Source: CAD feature listing. Evaluate the final solid. Frame: model axes, mm. A direction names the side the tool comes from. Round coordinates to 2 decimals unless told otherwise and drop trailing zeros. Loops run counter-clockwise (first coordinate to the right, second up) from the corner with the lowest first, then second, coordinate; pieces in that order, holes last. Notation, with made-up numbers: (80, -29.5) -> (88, -29.5) arc R17 ccw to (88, 2.5) -> close; hole circle Ø6 at (-29.75, 8). An arc over 180 degrees is marked (long way). Put each result on its own line as item: value. Start each with the question number.
1. Cut plane D-D (y = 216.5). Return the cut outline in (x, z) (3 decimals), then the cut area to 3 significant figures.
2. Set-up query: faces 1 (the flat face through (-104.51, 109.14, 1.57)), 2 (the flat face through (-156.49, 73.08, 1.57)). Return all of +Z, -Z, +X, -X, +Y, -Y with unobstructed straight access to the full face (end or side cutting, diameter ignored); none if empty.
3. Cut plane A-A (y = 186). Return the cut outline in (x, z) (3 decimals), then the cut area to 3 significant figures.
4. Cut plane C-C (x = -72.5). Return the cut outline in (y, z) (3 decimals), then the cut area to 3 significant figures.
5. Contact query for flat-ended pins moving along their axis: pin 1 (1.5 mm diameter, centred on x = 101, z = 1.5, fed in from +Y); pin 2 (1.7 mm diameter, centred on y = 231.5, z = 1.5, fed in from +X); pin 3 (1.6 mm diameter, centred on x = -182, z = 1.5, fed in from -Y). Output: stop coordinate, or through.
6. Material intervals for L1, parallel to X at y = 112.5, z = 0.85; L2, parallel to X at y = 188, z = 1.8; L3, parallel to Y at x = -52.5, z = 0.5, sorted ascending.
7. Cut plane B-B (y = 133). Return the cut outline in (x, z) (3 decimals).
```python
from build123d import *

# Parameters (mm, degrees)
BOSS_EXTRUDE1_DEPTH = 3.175
FILLET1_R           = 12.7
SKETCH3_W           = 50.8
SKETCH3_H           = 1.5875
BOSS_EXTRUDE2_DEPTH = 3.175
CUT_EXTRUDE1_DEPTH  = 305.700701144
CUT_EXTRUDE2_DEPTH  = 305.700701144
CUT_EXTRUDE3_REACH  = 306.045
SKETCH6_W           = 3.175
SKETCH6_H           = 11.1125
CUT_EXTRUDE5_START  = -3.175
CUT_EXTRUDE5_DEPTH  = 3.175
SKETCH8_W           = 471.002245988
SKETCH8_H           = 22.673608405
CUT_EXTRUDE6_DEPTH  = 305.045309672


with BuildPart() as part:
    # Sketch1 → Boss-Extrude1 (new body)
    with BuildSketch(Plane.XY):
        Polygon((-196.85, 0), (-63.5, 230.968975189), (63.5, 230.968975189), (196.85, 0), (167.520606325, 0), (48.835303163, 205.568975189), (-48.835303163, 205.568975189), (-167.520606325, 0), align=None)
    extrude(amount=BOSS_EXTRUDE1_DEPTH)

    # Fillet1
    fillet1_edges = [part.edges().sort_by_distance(p)[0] for p in [
        (167.520606325, 0, 1.5875),
        (48.835303163, 205.568975189, 1.5875),
        (-48.835303163, 205.568975189, 1.5875),
        (-167.520606325, 0, 1.5875),
    ]]
    fillet(fillet1_edges, radius=FILLET1_R)

    # Sketch3 → Boss-Extrude2 (add)
    with BuildSketch(Plane(origin=(0, 0, 0), x_dir=(-1, 0, 0), z_dir=(0, 0, -1))):
        Polygon((81.638815329, 202.726625451), (80.264, 201.932875451), (105.664, 157.938784939), (107.038815329, 158.732534939), align=None)
        Polygon((143.614815329, 95.381044601), (142.24, 94.587294601), (167.64, 50.593204089), (169.014815329, 51.386954089), align=None)
        with Locations((0, 231.762725189)):
            Rectangle(SKETCH3_W, SKETCH3_H)
    boss_extrude2 = extrude(amount=-BOSS_EXTRUDE2_DEPTH)

    # Sketch5 → Cut-Extrude1 (cut, through all)
    with BuildSketch(Plane(origin=(0, 0, 0), x_dir=(-1, 0, 0), z_dir=(0, 0, -1))):
        Polygon((-175.966912895, 19.672783942), (-185.491912895, 19.672783942), (-187.325, 16.497783942), (-186.309, 16.497783942), (-175.966912895, 16.497783942), align=None)
        Polygon((-186.309, 16.497783942), (-187.325, 16.497783942), (-196.85, 0), (-195.834, 0), align=None)
        Polygon((-121.132358029, 112.096802923), (-129.38125, 116.859302923), (-130.96875, 114.109672266), (-122.719858029, 109.347172266), align=None)
    cut_extrude1 = extrude(amount=-CUT_EXTRUDE1_DEPTH, mode=Mode.SUBTRACT)

    # Sketch4 → Cut-Extrude2 (cut, through all)
    with BuildSketch(Plane(origin=(0, 0, 0), x_dir=(-1, 0, 0), z_dir=(0, 0, -1))):
        Polygon((-61.666912895, 230.968975189), (-56.904412895, 222.720083218), (-59.654043552, 221.132583218), (-64.416543552, 229.381475189), (-63.5, 230.968975189), align=None)
    cut_extrude2 = extrude(amount=-CUT_EXTRUDE2_DEPTH, mode=Mode.SUBTRACT)

    # Mirror1: Boss-Extrude2, Cut-Extrude1, Cut-Extrude2 across plane
    add(boss_extrude2.mirror(Plane(origin=(0, 0, 0), x_dir=(0, 0, 1), z_dir=(1, 0, 0))))
    add(cut_extrude1.mirror(Plane(origin=(0, 0, 0), x_dir=(0, 0, 1), z_dir=(1, 0, 0))), mode=Mode.SUBTRACT)
    add(cut_extrude2.mirror(Plane(origin=(0, 0, 0), x_dir=(0, 0, 1), z_dir=(1, 0, 0))), mode=Mode.SUBTRACT)

    # Sketch6 → Cut-Extrude3 (cut, up to next)
    with BuildSketch(Plane(origin=(0, 0, 0), x_dir=(-1, 0, 0), z_dir=(0, 0, -1)), mode=Mode.PRIVATE) as cut_extrude3_sk1:
        with Locations((0, 227.000225189)):
            Rectangle(SKETCH6_W, SKETCH6_H)
    cut_extrude3_tool1 = extrude(cut_extrude3_sk1.sketch, amount=-CUT_EXTRUDE3_REACH, mode=Mode.PRIVATE) & part.part
    add(cut_extrude3_tool1.solids().sort_by_distance((0, 227.000225, 0))[0], mode=Mode.SUBTRACT)

    # Sketch7 → Cut-Extrude5 (cut)
    with BuildSketch(Plane(origin=(0, 0, 0), x_dir=(-1, 0, 0), z_dir=(0, 0, -1)).offset(CUT_EXTRUDE5_START)):
        Polygon((-61.666912895, 230.968975189), (-64.416543552, 229.381475189), (-62.698387042, 226.405540819), (-59.400779492, 228.178478093), (-60.980004947, 230.968975189), align=None)
        Polygon((-64.416543552, 229.381475189), (-64.498587563, 229.239370794), (-63.247784195, 226.110161009), (-62.698387042, 226.405540819), align=None)
        Polygon((64.498587563, 229.239370794), (63.247784195, 226.110161009), (59.400779492, 228.178478093), (60.980004947, 230.968975189), (61.666912895, 230.968975189), (64.416543552, 229.381475189), align=None)
    extrude(amount=CUT_EXTRUDE5_DEPTH, mode=Mode.SUBTRACT)

    # Sketch8 → Cut-Extrude6 (cut, through all)
    with BuildSketch(Plane(origin=(0, 0, 0), x_dir=(-1, 0, 0), z_dir=(0, 0, -1))):
        with Locations((-11.378610212, 5.16097974)):
            Rectangle(SKETCH8_W, SKETCH8_H)
    extrude(amount=-CUT_EXTRUDE6_DEPTH, mode=Mode.SUBTRACT)


solid = part.part
```
Solution:
1. outline: (-71.854, 0) -> (71.854, 0) -> (71.854, 3.175) -> (-71.854, 3.175) -> close
1. area: 456 mm^2
2. face 1: +Z, -Z, -Y
2. face 2: +Z, -Z, -X, +Y
3. outline: (-91.296, 0) -> (-60.133, 0) -> (-60.133, 3.175) -> (-91.296, 3.175) -> close; (60.133, 0) -> (91.296, 0) -> (91.296, 3.175) -> (60.133, 3.175) -> close
3. area: 198 mm^2
4. outline: (164.581, 0) -> (215.381, 0) -> (215.381, 3.175) -> (164.581, 3.175) -> close
4. area: 161 mm^2
5. pin 1: stops at y = 170.49
5. pin 2: stops at x = 60.98
5. pin 3: stops at y = 19.67
6. L1: x = -131.9 to -128.18, -121.83 to -102.57, 102.57 to 121.83, 128.18 to 131.9
6. L2: x = -90.14 to -58.98, 58.98 to 90.14
6. L3: y = 199.22 to 230.97
7. outline: (-120.062, 0) -> (-90.733, 0) -> (-90.733, 3.175) -> (-120.062, 3.175) -> close; (90.733, 0) -> (120.062, 0) -> (120.062, 3.175) -> (90.733, 3.175) -> close
